Job drawing, mm, ordinate dimensions from the low corner. One solid piece. A direction names the side the tool comes from. Give positions to 0.01 mm unless a question says otherwise; leave off trailing zeros. Write each loop counter-clockwise with the first axis right and the second up, starting at its lowest first coordinate (ties: lowest second). Pieces come first, ordered by that corner, then holes. Notation, with made-up numbers: M 27.5,0 L 66.5,0 A21 cw 66.5,7 Z; hole C 57.5,86.25 d10. An arc over 180 degrees is marked long. Answer as CSV lines item,"result". Start each with the question number.
Item 1: Two-plate mould, pull along Z, no slides. Class the marked faces 4, 5 and 6: +Z half, -Z half, draft (parallel to the pull), parting line (faces both ways), or undercut.
Item 2: 3-axis set-ups, long thin cutter, end or side, ignore diameter. For the marked faces 1, 2 and 3: which of +Z, -Z, +X, -X, +Y, -Y reach the whole face in a straight line?
Item 3: Band-saw the part on A-A, the plane y = 25. List the corners of the cut face in (x, z).
Item 4: Wall check: L1, parallel to Y at x = 80, z = 68; L2, parallel to Y at x = 20, z = 70; L3, parallel to Y at x = 7, z = 65.5. Give the ranges that are in metal, low to high. Write a range as from..to.
Item 5: Band-saw the part on B-B, the plane x = 20. List the corners of the cut face in (y, z), then the cut area to 3 significant figures.
Item 6: Pin check, flat tips, straight feed: pin 1 (2 mm diameter, centred on x = 41, z = 39.5, fed in from +Y); pin 2 (3 mm diameter, centred on x = 55.5, y = 58, fed in from -Z); pin 3 (0.6 mm diameter, centred on x = 30, z = 1, fed in from +Y); pin 4 (8 mm diameter, centred on x = 20, y = 25, fed in from -Z). Stop position of each tip, or through.
Item 7: Band-saw the part on C-C, the plane x = 87. List the corners of the cut face in (y, z).
Item 8: Band-saw the part on D-D, the plane y = 33.5. List the corners of the cut face in (x, z), then the cut area to 3 significant figures.
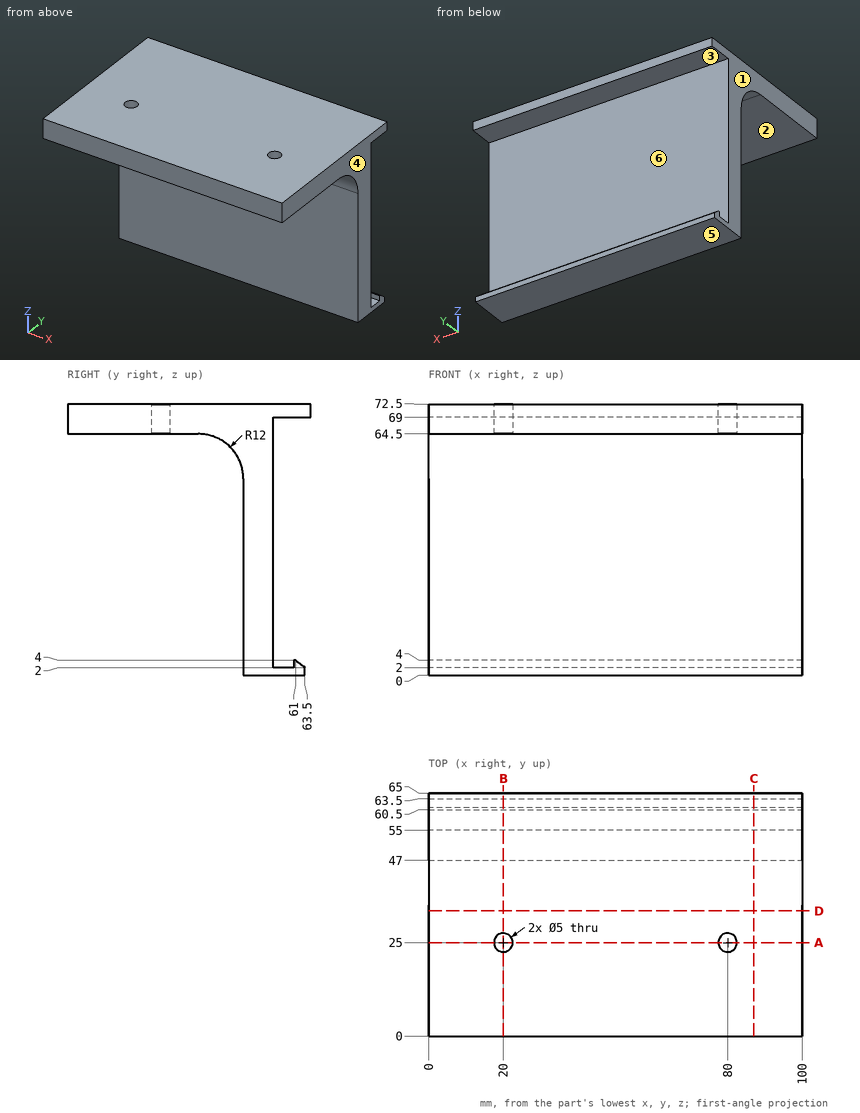
Output:
1,face 4,"draft"
1,face 5,"-Z half"
1,face 6,"undercut"
2,face 1,"+Z, -Z, -X, +Y, -Y"
2,face 2,"-Z, +X, -X, -Y"
2,face 3,"+X, -X, +Y"
3,outline,"M 0,64.5 L 17.5,64.5 L 17.5,72.5 L 0,72.5 Z; M 22.5,64.5 L 77.5,64.5 L 77.5,72.5 L 22.5,72.5 Z; M 82.5,64.5 L 100,64.5 L 100,72.5 L 82.5,72.5 Z"
4,L1,"0..22.5, 27.5..55"
4,L2,"0..22.5, 27.5..65"
4,L3,"0..55"
5,outline,"M 0,64.5 L 22.5,64.5 L 22.5,72.5 L 0,72.5 Z; M 27.5,64.5 L 35,64.5 A12 cw 47,52.5 L 47,0 L 63.5,0 L 63.5,2 L 61,4 L 60.5,4 L 60.5,2 L 55,2 L 55,69 L 65,69 L 65,72.5 L 27.5,72.5 Z"
5,area,"1,000 mm²"
6,pin 1,"y = 55"
6,pin 2,"z = 0"
6,pin 3,"y = 63.5"
6,pin 4,"z = 64.5"
7,outline,"M 0,64.5 L 35,64.5 A12 cw 47,52.5 L 47,0 L 63.5,0 L 63.5,2 L 61,4 L 60.5,4 L 60.5,2 L 55,2 L 55,69 L 65,69 L 65,72.5 L 0,72.5 Z"
8,outline,"M 0,64.5 L 100,64.5 L 100,72.5 L 0,72.5 Z"
8,area,"800 mm²"
